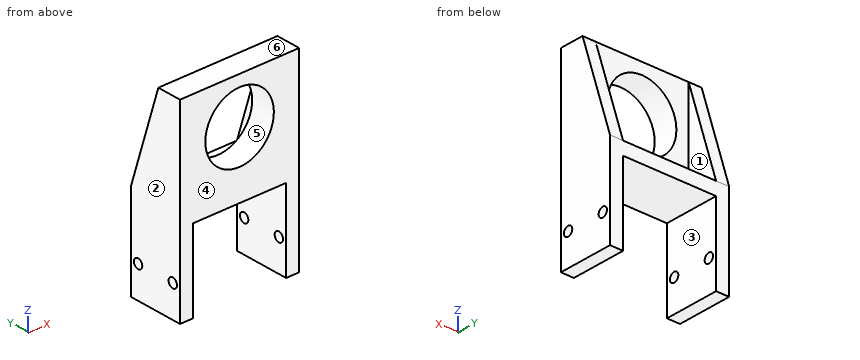
from build123d import *

# Parameters (mm, degrees)
BOSS_EXTRUDE1_DEPTH            = 17
M2_5_START                     = -4
M2_5_CLEARANCE_HOLE1_OUTLINE_R = 1.45
M2_5_CLEARANCE_HOLE1_DEPTH     = 36.5
SKETCH6_W                      = 36.5
SKETCH6_H                      = 17
BOSS_EXTRUDE2_DEPTH            = 30
SKETCH7_R                      = 10.5
CUT_EXTRUDE1_DEPTH             = 51.012498438
SKETCH8_W                      = 36.5
SKETCH8_H                      = 30
CUT_EXTRUDE2_DEPTH             = 9.5
RIB1_REACH                     = 54.7
SKETCH9_WALL_W                 = 138.86747894
SKETCH9_WALL_H                 = 4
RIB2_START                     = -4
RIB2_DEPTH                     = 4


# Read off the part's stored shape, not the designer's step: M2.5 Clearance Hole1, Rib2
with BuildPart() as part:
    # Sketch1 → Boss-Extrude1 (new body)
    with BuildSketch(Plane(origin=(0, 0, 0), x_dir=(1, 0, 0), z_dir=(0, 1, 0))):
        Polygon((32.5, -4), (32.5, 25), (28.5, 25), (28.5, 0), (0, 0), (0, 25), (-4, 25), (-4, -4), align=None)
    extrude(amount=BOSS_EXTRUDE1_DEPTH)

    # M2.5 Clearance Hole1 outline → M2.5 Clearance Hole1 (cut)
    with BuildSketch(Plane.YZ.offset(M2_5_START)):
        with Locations((2.5, -15.25)):
            Circle(M2_5_CLEARANCE_HOLE1_OUTLINE_R)
        with Locations((14.5, -15.25)):
            Circle(M2_5_CLEARANCE_HOLE1_OUTLINE_R)
    extrude(amount=M2_5_CLEARANCE_HOLE1_DEPTH, mode=Mode.SUBTRACT)

    # Sketch6 → Boss-Extrude2 (add)
    with BuildSketch(Plane.XY.offset(4)):
        with Locations((14.25, 8.5)):
            Rectangle(SKETCH6_W, SKETCH6_H)
    extrude(amount=BOSS_EXTRUDE2_DEPTH)

    # Sketch7 → Cut-Extrude1 (cut, through all)
    with BuildSketch(Plane(origin=(0, 17, 0), x_dir=(1, 0, 0), z_dir=(0, 1, 0))):
        with Locations(Location((14.25, -20, 0), (0, 0, 270))):
            Circle(SKETCH7_R)
    extrude(amount=-CUT_EXTRUDE1_DEPTH, mode=Mode.SUBTRACT)

    # Sketch8 → Cut-Extrude2 (cut)
    with BuildSketch(Plane(origin=(0, 17, 0), x_dir=(1, 0, 0), z_dir=(0, 1, 0))):
        with Locations((14.25, -19)):
            Rectangle(SKETCH8_W, SKETCH8_H)
    extrude(amount=-CUT_EXTRUDE2_DEPTH, mode=Mode.SUBTRACT)

    # Sketch9 wall → Rib1 (add, up to next)
    with BuildSketch(Plane(origin=(32.5, 12.25, 19), x_dir=(0, 0.301891704694, -0.953342225351), z_dir=(0, 0.953342225351, 0.301891704694)), mode=Mode.PRIVATE) as rib1_sk1:
        with Locations((0, 2)):
            Rectangle(SKETCH9_WALL_W, SKETCH9_WALL_H)
    rib1_tool1 = extrude(rib1_sk1.sketch, amount=-RIB1_REACH, mode=Mode.PRIVATE) - part.part
    add(rib1_tool1.solids().sort_by_distance((32.5, 12.25, 19))[0])

    # Rib2 outline → Rib2 (add)
    with BuildSketch(Plane.ZY.offset(4).offset(RIB2_START)):
        Polygon((34, 7.5), (4, 17), (4, 7.5), align=None)
    extrude(amount=RIB2_DEPTH)


solid = part.part
The listing builds one solid part. Answer for the finished solid, in the listing's coordinates (mm). Face numbers are marked on the shaded views. A direction names the side the tool comes from. Round coordinates to 2 decimals unless told otherwise and drop trailing zeros. Write each loop counter-clockwise with the first axis right and the second up, starting at its lowest first coordinate (ties: lowest second). Pieces come first, ordered by that corner, then holes. Notation, with made-up numbers: (31, -3.5) - (36, -3.5) arc R18 cw to (36, 26.5) - close; hole circle Ø9 at (-22.75, 39). An arc over 180 degrees is marked (long way). Use one line per item in the form item = value. Start each with the question number.
Item 1: A cutting plane is placed at D-D (z = -6). Write down the section's boundary in (x, y), plus the area to 3 significant figures.
Item 2: Find the intervals of material crossed by line 1 (Y direction, x = 30.5, z = -15.25); line 2 (X direction, y = 5.75, z = 20); line 3 (X direction, y = 9, z = -17.5), in increasing order. Write a range as [from, to].
Item 3: Flat-ended cylindrical pins translate along their axes: pin 1 Ø1.7 at (y, z) = (14.5, -15.25) entering from +X; pin 2 Ø6 at (x, y) = (7, 9) entering from -Z; pin 3 Ø1.5 at (x, y) = (8.5, 12) entering from +Z. Find the tip coordinate at first contact, or state that the pin passes through.
Item 4: Determine the mould class of the marked faces 4, 5 and 6 for opening direction Z: +Z half, -Z half, draft (parallel to the pull), parting line (faces both ways), or undercut.
Item 5: A tool of negligible diameter and unlimited length cuts with its end or side. For the marked faces 1, 2 and 3, from which of +Z, -Z, +X, -X, +Y, -Y can it reach the whole face along a straight path? Write none if from no direction.
Item 6: A cutting plane is placed at A-A (z = -15.25). Write down the section's boundary in (x, y), plus the area to 3 significant figures.
Item 7: A cutting plane is placed at C-C (x = 17). Write down the section's boundary in (y, z).
Item 8: A cutting plane is placed at B-B (y = 5). Write down the section's boundary in (x, z), plus the area to 3 significant figures.
The answers:
q1.outline = (-4, 0) - (0, 0) - (0, 17) - (-4, 17) - close; (28.5, 0) - (32.5, 0) - (32.5, 17) - (28.5, 17) - close
q1.area = 136 mm^2
q2.line_1 = [0, 1.05], [3.95, 13.05], [15.95, 17]
q2.line_2 = [-4, 3.75], [24.75, 32.5]
q2.line_3 = [-4, 0], [28.5, 32.5]
q3.pin_1 = through
q3.pin_2 = 0
q3.pin_3 = 4
q4.face_4 = draft
q4.face_5 = undercut
q4.face_6 = +Z half
q5.face_1 = +Z, +Y
q5.face_2 = +Z, -Z, -X, +Y, -Y
q5.face_3 = -Z, +Y, -Y
q6.outline = (-4, 0) - (0, 0) - (0, 1.05) - (-4, 1.05) - close; (-4, 3.95) - (0, 3.95) - (0, 13.05) - (-4, 13.05) - close; (-4, 15.95) - (0, 15.95) - (0, 17) - (-4, 17) - close; (28.5, 0) - (32.5, 0) - (32.5, 1.05) - (28.5, 1.05) - close; (28.5, 3.95) - (32.5, 3.95) - (32.5, 13.05) - (28.5, 13.05) - close; (28.5, 15.95) - (32.5, 15.95) - (32.5, 17) - (28.5, 17) - close
q6.area = 89.6 mm^2
q7.outline = (0, 0) - (17, 0) - (17, 4) - (7.5, 4) - (7.5, 9.87) - (0, 9.87) - close; (0, 30.13) - (7.5, 30.13) - (7.5, 34) - (0, 34) - close
q8.outline = (-4, -25) - (0, -25) - (0, 0) - (28.5, 0) - (28.5, -25) - (32.5, -25) - (32.5, 34) - (-4, 34) - close; hole circle Ø21 at (14.25, 20)
q8.area = 1,090 mm^2
